Source: CAD feature listing. Evaluate the final solid. Frame: model axes, mm. A direction names the side the tool comes from. Give positions to 0.01 mm unless a question says otherwise; leave off trailing zeros. Loops run counter-clockwise (first coordinate to the right, second up) from the corner with the lowest first, then second, coordinate; pieces in that order, holes last. Notation, with made-up numbers: (65, 48) -> (106, 48) arc R27 cw to (106, 79) -> close; hole circle Ø2 at (83.5, 35). An arc over 180 degrees is marked (long way). Return JSON: item names as keys, results as strings. Group by question number.
```python
from build123d import *

# Parameters (mm, degrees)
SKETCH1_R               = 15.875
BOSS_EXTRUDE1_DEPTH     = 4.826
CUT_EXTRUDE1_DEPTH      = 25.437519391
CUT_EXTRUDE2_DEPTH      = 25.437519391
CUT_EXTRUDE3_DEPTH      = 23.963482445
CUT_EXTRUDE3_DEPTH_BACK = 23.963482445
SKETCH4_R               = 2.3876


with BuildPart() as part:
    # Sketch1 → Boss-Extrude1 (new, symmetric)
    with BuildSketch(Plane.XY):
        Circle(SKETCH1_R)
    extrude(amount=BOSS_EXTRUDE1_DEPTH, both=True)

    # Sketch2 → Cut-Extrude1 (cut, through all)
    with BuildSketch(Plane.XY.offset(4.826)):
        Polygon((-6.4135, 3.702835951), (-6.4135, -3.702835951), (0, -7.405671903), (6.4135, -3.702835951), (6.4135, 3.702835951), (0, 7.405671903), align=None)
    extrude(amount=-CUT_EXTRUDE1_DEPTH, mode=Mode.SUBTRACT)

    # Sketch3 → Cut-Extrude2 (cut, through all)
    with BuildSketch(Plane.XY.offset(4.826)):
        with BuildLine():
            Line((-15.870427341, 0.381), (12.7, 0.381))
            Line((12.7, 0.381), (12.7, -0.381))
            Line((12.7, -0.381), (-15.870427341, -0.381))
            ThreePointArc((-15.870427341, -0.381), (-15.875, 0), (-15.870427341, 0.381))
        make_face()
    extrude(amount=-CUT_EXTRUDE2_DEPTH, mode=Mode.SUBTRACT)

    # Sketch4 → Cut-Extrude3 (cut, two sides: drawn at the far end of the back side and taken through both)
    with BuildSketch(Plane(origin=(0, 0, 0), x_dir=(1, 0, 0), z_dir=(0, 1, 0)).offset(-CUT_EXTRUDE3_DEPTH_BACK)):
        with Locations(Location((-11.044427341, 0, 0), (0, 0, 270))):
            Circle(SKETCH4_R)
    extrude(amount=CUT_EXTRUDE3_DEPTH + CUT_EXTRUDE3_DEPTH_BACK, mode=Mode.SUBTRACT)


solid = part.part
```
1) Mould query, pull axis Z, two halves, no side actions, for faces 4 (the face through (3, -7, 4.826)), 5 (the face through (-8.677, -5.498, -0.311)), 6 (the face through (3.3, 5.5, 0.1)). Classes: released by +Z, released by -Z, zero draft, split by the parting line, or undercut.
2) Cut plane D-D on x = -9.5. Return loops of the section in (y, z), then the cut area to 3 significant figures.
3) Cut plane A-A on x = 6. Return loops of the section in (y, z), then the cut area to 3 significant figures.
4) Cut plane B-B on z = 0.25. Count the separate pieces of the cut face and the enclosed holes in it, then the cut area to 3 significant figures.
5) Contact query for flat-ended pins moving along their axis: P1, Ø2.5, axis at y = -2.5, z = -2, coming from the -X side; P2, Ø1, axis at y = -1.5, z = 2, coming from the +X side; P3, Ø4, axis at x = 10.5, z = -3.5, coming from the +Y side; P4, Ø4.5, axis at x = -11.04, z = 0, coming from the +Y side. Output: stop coordinate, or through.
6) Cut plane C-C on y = -1. Return loops of the section in (x, z), then the cut area to 3 significant figures.
7) Reachability of faces 1 (the face through (-3.3, -5.5, 0.1)), 2 (the face through (-8.677, 5.317, -0.311)), 3 (the face through (10, 0.381, 0)) from +Z, -Z, +X, -X, +Y, -Y: full face, straight path, thin tool, end or side. Return the list, or none.
8) Material intervals for line 1 (X direction, y = -3.5, z = 0); line 2 (X direction, y = -6, z = 0); line 3 (Y direction, x = -12, z = 3.25), sorted ascending.
Calculated:
{
 "1": {"face 4": "released by +Z", "face 5": "undercut", "face 6": "zero draft"},
 "2": {"outline": "(-12.72, -4.83) -> (-0.38, -4.83) -> (-0.38, -1.82) -> (-12.72, -1.82) -> close; (-12.72, 1.82) -> (-0.38, 1.82) -> (-0.38, 4.83) -> (-12.72, 4.83) -> close; (0.38, -4.83) -> (12.72, -4.83) -> (12.72, -1.82) -> (0.38, -1.82) -> close; (0.38, 1.82) -> (12.72, 1.82) -> (12.72, 4.83) -> (0.38, 4.83) -> close", "area": "148 mm2"},
 "3": {"outline": "(-14.7, -4.83) -> (-3.94, -4.83) -> (-3.94, 4.83) -> (-14.7, 4.83) -> close; (3.94, -4.83) -> (14.7, -4.83) -> (14.7, 4.83) -> (3.94, 4.83) -> close", "area": "208 mm2"},
 "4": {"separate pieces": "3", "enclosed holes": "0", "area": "534 mm2"},
 "5": {"P1": "x = -15.83", "P2": "x = 15.84", "P3": "y = 13.41", "P4": "through"},
 "6": {"outline": "(-15.84, -4.83) -> (-6.41, -4.83) -> (-6.41, 4.83) -> (-15.84, 4.83) -> close; (6.41, -4.83) -> (15.84, -4.83) -> (15.84, 4.83) -> (6.41, 4.83) -> close; hole circle Ø4.78 at (-11.04, 0)", "area": "164 mm2"},
 "7": {"face 1": "+Z, -Z", "face 2": "+Y, -Y", "face 3": "+Z, -Z, -X"},
 "8": {"line 1": "-15.48 to -13.43, -8.66 to -6.41, 6.41 to 15.48", "line 2": "-14.7 to -13.43, -8.66 to -2.43, 2.43 to 14.7", "line 3": "-10.39 to -0.38, 0.38 to 10.39"}
}
